Geometry: final body of the model. Coordinates: model frame, mm. Face numbers are marked on the shaded views. Coordinates: 2 decimals unless noted, no trailing zeros. Order: outer loops, then holes, each group sorted by start corner. A loop starts at its lowest first (then second) coordinate and runs counter-clockwise, first axis right, second up. Notation, with made-up numbers: (18, 18) -> (31, 18) arc R13 cw to (31, 30) -> close; hole circle Ø5 at (50.5, -16.5). An arc over 180 degrees is marked (long way). Use one line per item in the form item = value.
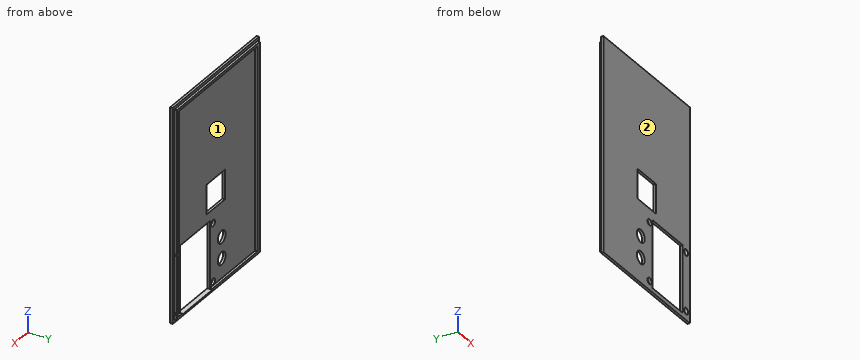
```python
from build123d import *

# Parameters (mm, degrees)
SKETCH1_W           = 55.5
SKETCH1_H           = 85.5
BOSS_EXTRUDE1_DEPTH = 1
SKETCH2_W           = 53.25
SKETCH2_H           = 83.25
SKETCH2_W_2         = 50.3558552
SKETCH2_H_2         = 81.260119932
BOSS_EXTRUDE2_DEPTH = 1
SKETCH3_R           = 2.5
SKETCH3_R_2         = 1.25
SKETCH3_R_3         = 1.248818361
SKETCH3_R_4         = 1.252029075
SKETCH3_W           = 19.3
SKETCH3_H           = 26.9
SKETCH3_W_2         = 11.8
SKETCH3_H_2         = 11.8
CUT_EXTRUDE2_DEPTH  = 3


with BuildPart() as part:
    # Sketch1 → Boss-Extrude1 (new body)
    with BuildSketch(Plane(origin=(0, 0, 0), x_dir=(1, 0, 0), z_dir=(0, 1, 0))):
        Rectangle(SKETCH1_W, SKETCH1_H)
    extrude(amount=BOSS_EXTRUDE1_DEPTH)

    # Sketch2 → Boss-Extrude2 (add)
    with BuildSketch(Plane(origin=(0, 1, 0), x_dir=(1, 0, 0), z_dir=(0, 1, 0))):
        Rectangle(SKETCH2_W, SKETCH2_H)
        Rectangle(SKETCH2_W_2, SKETCH2_H_2, mode=Mode.SUBTRACT)
    extrude(amount=BOSS_EXTRUDE2_DEPTH)

    # Sketch3 → Cut-Extrude2 (cut)
    with BuildSketch(Plane.XZ):
        with Locations(Location((-3.75, -32.75, 0), (0, 0, 270))):
            Circle(SKETCH3_R)
        with Locations(Location((-3.75, -24.25, 0), (0, 0, 270))):
            Circle(SKETCH3_R)
        with Locations(Location((1.819004369, -15.96241079, 0), (0, 0, 270))):
            Circle(SKETCH3_R_2)
        with Locations(Location((25.419004357, -15.963142334, 0), (0, 0, 270))):
            Circle(SKETCH3_R_3)
        with Locations(Location((1.818587591, -39.162410787, 0), (0, 0, 270))):
            Circle(SKETCH3_R_2)
        with Locations(Location((25.419004357, -39.162410787, 0), (0, 0, 270))):
            Circle(SKETCH3_R_4)
        with Locations((13.569004369, -27.574665711)):
            Rectangle(SKETCH3_W, SKETCH3_H)
        with Locations((0.091347466, -4.575788212)):
            Rectangle(SKETCH3_W_2, SKETCH3_H_2)
    extrude(amount=-CUT_EXTRUDE2_DEPTH, mode=Mode.SUBTRACT)


solid = part.part
```
1) Section D-D, the plane z = 9.5. Output: boundary loops of the cut face in (x, y) (3 decimals).
Results found:
outline = (-27.75, 0) -> (27.75, 0) -> (27.75, 1) -> (26.625, 1) -> (26.625, 2) -> (25.178, 2) -> (25.178, 1) -> (-25.178, 1) -> (-25.178, 2) -> (-26.625, 2) -> (-26.625, 1) -> (-27.75, 1) -> close
2) Material intervals for probe 1 along Z at (x, y) = (5, 0.1); probe 2 along X at (y, z) = (1.5, -37) (3 decimals); probe 3 along X at (y, z) = (0.4, -24.25), sorted ascending. Write a range as from..to.
Results found:
probe_1 = -42.75..-41.02, -14.12..-10.48, 1.32..42.75
probe_2 = -26.625..-25.178, 25.178..26.625
probe_3 = -27.75..-6.25, -1.25..3.92, 23.22..27.75
3) Section C-C, the plane z = -32.75. Output: boundary loops of the cut face in (x, y) (3 decimals).
Results found:
outline = (-27.75, 0) -> (-6.25, 0) -> (-6.25, 1) -> (-25.178, 1) -> (-25.178, 2) -> (-26.625, 2) -> (-26.625, 1) -> (-27.75, 1) -> close; (-1.25, 0) -> (3.919, 0) -> (3.919, 1) -> (-1.25, 1) -> close; (23.219, 0) -> (27.75, 0) -> (27.75, 1) -> (26.625, 1) -> (26.625, 2) -> (25.178, 2) -> (25.178, 1) -> (23.219, 1) -> close
4) Section B-B, the plane x = -3.75. Output: boundary loops of the cut face in (y, z) (3 decimals).
Results found:
outline = (0, -42.75) -> (1, -42.75) -> (1, -41.625) -> (2, -41.625) -> (2, -40.63) -> (1, -40.63) -> (1, -35.25) -> (0, -35.25) -> close; (0, -30.25) -> (1, -30.25) -> (1, -26.75) -> (0, -26.75) -> close; (0, -21.75) -> (1, -21.75) -> (1, -10.476) -> (0, -10.476) -> close; (0, 1.324) -> (1, 1.324) -> (1, 40.63) -> (2, 40.63) -> (2, 41.625) -> (1, 41.625) -> (1, 42.75) -> (0, 42.75) -> close
5) Contact query for flat-ended pins moving along their axis: P1, Ø0.5, axis at y = 1.5, z = -29.5, coming from the -X side (3 decimals); P2, Ø6, axis at x = -3.75, z = -24.25, coming from the +Y side; P3, Ø2, axis at x = 1.82, z = -39.16, coming from the +Y side. Output: stop coordinate, or through.
Results found:
P1 = -26.625
P2 = 1
P3 = through
6) Section A-A, the plane x = 19. Output: boundary loops of the cut face in (y, z) (3 decimals), and give its area (3 significant figures).
Results found:
outline = (0, -42.75) -> (1, -42.75) -> (1, -41.625) -> (2, -41.625) -> (2, -41.025) -> (0, -41.025) -> close; (0, -14.125) -> (1, -14.125) -> (1, 40.63) -> (2, 40.63) -> (2, 41.625) -> (1, 41.625) -> (1, 42.75) -> (0, 42.75) -> close
area = 60.2 mm2
7) Pull-direction query (Z, two-part tool) for the marked faces 1 and 2; classes: released by +Z, released by -Z, zero draft, split by the parting line, or undercut.
Results found:
face_1 = undercut
face_2 = zero draft
